Design review of the part built by this model. Coordinates are the model's own, in mm. Round coordinates to 2 decimals unless told otherwise and drop trailing zeros. One line per question, with ' | ' between items. Start each with the question number.
1) Mouldability with a two-part tool opening along Y and no side actions: class faces 1 (the flat face through (-63, 2, 4)), 2 (the cylindrical face through (-15.803, 0.878, 1.972)) as +Y half, -Y half, draft (parallel to the pull), parting line (faces both ways), or undercut.
2) Insertion check: pin 1 Ø5.5 at (x, y) = (-100, -160.44) entering from +Z. The pin has a flat end and moves straight along its axis. Give the tip position at first contact, or say it passes through.
3) For probe 1 along Y at (x, z) = (0, 1.1); probe 2 along Y at (x, z) = (60, 2.6); probe 3 along Y at (x, z) = (-97.5, 0.9), list the stretches that pass through material, from the lowest coordinate up.
```python
from build123d import *

# Parameters (mm, degrees)
SKETCH_1_W          = 360
SKETCH_1_H          = 360
SKETCH_1_R          = 2
SKETCH_1_R_2        = 4.4
EXTRUDE_1_DEPTH     = 4
SKETCH_2_R          = 1.5
CUT_EXTRUDE_2_DEPTH = 20
SKETCH_3_R          = 3.04
CUT_EXTRUDE_3_DEPTH = 20


with BuildPart() as part:
    # 草图1 → 凸台-拉伸1 (new body)
    with BuildSketch(Plane.XY):
        with Locations((-20, -0.443736876)):
            Rectangle(SKETCH_1_W, SKETCH_1_H)
        with Locations((-40, -0.443736876)):
            Circle(SKETCH_1_R, mode=Mode.SUBTRACT)
        with Locations((-40, 39.556263124)):
            Circle(SKETCH_1_R, mode=Mode.SUBTRACT)
        with Locations((0, 39.556263124)):
            Circle(SKETCH_1_R, mode=Mode.SUBTRACT)
        with Locations((0, -0.443736876)):
            Circle(SKETCH_1_R, mode=Mode.SUBTRACT)
        with Locations(Location((0, -40.443736876, 0), (0, 0, 180))):
            Circle(SKETCH_1_R, mode=Mode.SUBTRACT)
        with Locations(Location((-40, -40.443736876, 0), (0, 0, 180))):
            Circle(SKETCH_1_R, mode=Mode.SUBTRACT)
        with Locations((-20, -0.443736876)):
            Circle(SKETCH_1_R_2, mode=Mode.SUBTRACT)
    extrude(amount=EXTRUDE_1_DEPTH)

    # 草图2 → 切除-拉伸2 (cut)
    with BuildSketch(Plane.XY.offset(4)):
        with Locations((57.061153948, -42.313752709)):
            Circle(SKETCH_2_R)
        with Locations((84.961153948, -42.313752709)):
            Circle(SKETCH_2_R)
        with Locations((44.561153948, -93.113752709)):
            Circle(SKETCH_2_R)
        with Locations((90.061153948, -94.413752709)):
            Circle(SKETCH_2_R)
        with Locations((40.061153948, 24.768466173)):
            Circle(SKETCH_2_R)
        with Locations((89.061153948, 24.768466173)):
            Circle(SKETCH_2_R)
        with Locations((40.061153948, -33.231533827)):
            Circle(SKETCH_2_R)
        with Locations((89.061153948, -33.231533827)):
            Circle(SKETCH_2_R)
    extrude(amount=-CUT_EXTRUDE_2_DEPTH, mode=Mode.SUBTRACT)

    # 草图3 → 切除-拉伸3 (cut)
    with BuildSketch(Plane.XY.offset(4)):
        with Locations((-180, -160.443736876)):
            Circle(SKETCH_3_R)
        with Locations((-180, -80.443736876)):
            Circle(SKETCH_3_R)
        with Locations((-180, -0.443736876)):
            Circle(SKETCH_3_R)
        with Locations((-180, 79.556263124)):
            Circle(SKETCH_3_R)
        with Locations((-180, 159.556263124)):
            Circle(SKETCH_3_R)
        with Locations((-100, 159.556263124)):
            Circle(SKETCH_3_R)
        with Locations((-20, 159.556263124)):
            Circle(SKETCH_3_R)
        with Locations((60, 159.556263124)):
            Circle(SKETCH_3_R)
        with Locations((140, 159.556263124)):
            Circle(SKETCH_3_R)
        with Locations((140, 79.556263124)):
            Circle(SKETCH_3_R)
        with Locations((140, -0.443736876)):
            Circle(SKETCH_3_R)
        with Locations((140, -80.443736876)):
            Circle(SKETCH_3_R)
        with Locations((140, -160.443736876)):
            Circle(SKETCH_3_R)
        with Locations((60, -160.443736876)):
            Circle(SKETCH_3_R)
        with Locations((-20, -160.443736876)):
            Circle(SKETCH_3_R)
        with Locations((-100, -160.443736876)):
            Circle(SKETCH_3_R)
    extrude(amount=-CUT_EXTRUDE_3_DEPTH, mode=Mode.SUBTRACT)


solid = part.part
```
From the geometry:
1) face 1: draft | face 2: undercut
2) pin 1: passes through
3) probe 1: y = -180.44 to -42.44, -38.44 to -2.44, 1.56 to 37.56, 41.56 to 179.56 | probe 2: y = -180.44 to -163.48, -157.4 to 156.52, 162.6 to 179.56 | probe 3: y = -180.44 to -162.17, -158.71 to 157.83, 161.29 to 179.56
